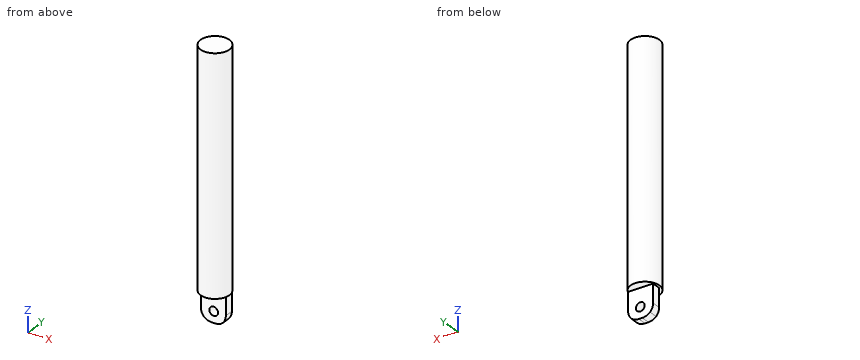
from build123d import *

# Parameters (mm, degrees)
SKETCH1_W           = 80
SKETCH1_H           = 4.95
SKETCH2_W           = 8.501628875
SKETCH2_H           = 3.058191312
BOSS_EXTRUDE1_DEPTH = 50
CHAMFER1_SIZE       = 2
FILLET1_R           = 4
HOLE1_START         = -3.599264013
HOLE1_OUTLINE_R     = 1.5
HOLE1_DEPTH         = 3.058191312
SCALE1_SCALE        = 18.33


# Read off the part's stored shape, not the designer's step: Hole1
with BuildPart() as part:
    # Sketch1 → Revolve1 (revolve)
    with BuildSketch(Plane(origin=(0, 0, 0), x_dir=(0, 0, -1), z_dir=(1, 0, 0))):
        Rectangle(SKETCH1_W, SKETCH1_H)
    revolve(axis=Axis((0, -2.475, -40), (0, 0, 1)))

    # Sketch2 → Boss-Extrude1 (add)
    with BuildSketch(Plane.XY):
        with Locations((0.196159038, -2.070168357)):
            Rectangle(SKETCH2_W, SKETCH2_H)
    extrude(amount=-BOSS_EXTRUDE1_DEPTH)

    # Chamfer1
    chamfer1_edges = [part.edges().sort_by_distance(p)[0] for p in [
        (4.446973476, -2.070168357, -50),
        (-4.054655399, -2.070168357, -50),
    ]]
    chamfer(chamfer1_edges, length=CHAMFER1_SIZE)

    # Fillet1
    # the kernel refuses this fillet: 4 mm, written as the material it takes off along each edge
    with BuildSketch(Plane(origin=(-2.054655399, 3.601062923, -50), x_dir=(-0.7071067811865491, 0, 0.7071067811865459), z_dir=(0, -1, 0)), Plane(origin=(4.446973476, -7.741399637, -48), x_dir=(0, 0, 1), z_dir=(0, 1, 0)), Plane(origin=(-4.054655399, 3.601062923, -48), x_dir=(0, 0, 1), z_dir=(0, -1, 0))) as fillet1_piece_1:
        with BuildLine():
            CenterArc((FILLET1_R * 0.414213562373, -FILLET1_R), FILLET1_R, 90, 45)
            Line((-FILLET1_R * 0.292893218813, -FILLET1_R * 0.292893218813), (0, 0))
            Line((0, 0), (FILLET1_R * 0.414213562373, 0))
        make_face()
    extrude(amount=11.34246256, mode=Mode.SUBTRACT)
    with BuildSketch(Plane(origin=(2.446973476, -7.741399637, -50), x_dir=(-1, 0, 0), z_dir=(0, 1, 0))) as fillet1_piece_2:
        with BuildLine():
            CenterArc((FILLET1_R * 0.414213562373, FILLET1_R), FILLET1_R, 225, 45)
            Line((-FILLET1_R * 0.292893218813, FILLET1_R * 0.292893218813), (0, 0))
            Line((0, 0), (FILLET1_R * 0.414213562373, 0))
        make_face()
    extrude(amount=11.34246256, mode=Mode.SUBTRACT)

    # Hole1 outline → Hole1 (cut)
    with BuildSketch(Plane(origin=(0, 0, 0), x_dir=(1, 0, 0), z_dir=(0, 1, 0)).offset(HOLE1_START)):
        with Locations((0.316437215, 46.206035657)):
            Circle(HOLE1_OUTLINE_R)
    extrude(amount=HOLE1_DEPTH, mode=Mode.SUBTRACT)


with BuildPart() as part_1:
    # Scale1: scaled about (0.006416206, -2.460917228, -1.550485335)
    add(part.part.scale(SCALE1_SCALE).moved(Location((-0.11119285, 42.647695561, 26.869910856))))


solid = part_1.part
Can you work these out from the model? Positions are in its coordinate system, mm. Round coordinates to 2 decimals unless told otherwise and drop trailing zeros. Loops run counter-clockwise (first coordinate to the right, second up) from the corner with the lowest first, then second, coordinate; pieces in that order, holes last. Notation, with made-up numbers: (-13.5, 23) - (20.5, 23) arc R10 cw to (20.5, 38) - close; hole circle Ø6 at (33.5, -34.75). An arc over 180 degrees is marked (long way). Answer in a Markdown table with one row per item. Add a question column.
Q1. I want a section at D-D on z = -276.5. List the corners of the cut face in (x, y) for me.
Q2. I want a section at C-C on y = -57. List the corners of the cut face in (x, z) for me.
Q3. For pin 1 Ø10 at (x, z) = (-72, -262) entering from -Y; pin 2 Ø1.5 at (x, y) = (39.5, -44) entering from -Z; pin 3 Ø1.5 at (x, z) = (45, 363) entering from +Y, each with a flat end and sliding along its axis, tell me the tip position at first contact or that it passes through.
Q4. I want a section at B-B on x = -42. List the corners of the cut face in (y, z) for me, and give its area (3 significant figures).
Q5. I need wall thicknesses on L1, parallel to Z at x = 3, y = 21; L2, parallel to Z at x = 1.5, y = -11.5; L3, parallel to Z at x = 37.5, y = -27. Which ranges of each line are inside material? Lowest first, please.
Q6. I want a section at A-A on y = 7.5. List the corners of the cut face in (x, z) for me (3 decimals), and give its area (3 significant figures).
A:
| question | item | result |
|---|---|---|
| 1 | outline | circle Ø181.47 at (-0.11, -2.72) |
| 2 | outline | (-72.82, -706.33) - (72.59, -706.33) - (72.59, 760.07) - (-72.82, 760.07) - close |
| 3 | pin 1 | y = -64.03 |
| 3 | pin 2 | z = -706.33 |
| 3 | pin 3 | y = 76.43 |
| 4 | outline | (-83.2, -706.33) - (-23.33, -706.33) - (-23.33, -880.95) - (32.73, -880.95) - (32.73, -706.33) - (77.77, -706.33) - (77.77, 760.07) - (-83.2, 760.07) - close |
| 4 | area | 246,000 mm^2 |
| 5 | L1 | -889.63 to -847.45, -792.72 to 760.07 |
| 5 | L2 | -889.63 to -847.26, -792.91 to 760.07 |
| 5 | L3 | -706.33 to 760.07 |
| 6 | outline | (-90.267, -706.33) - (-74.433, -706.33) - (-74.433, -822.6) arc R73.32 ccw to (-56.008, -871.205) arc R73.32 ccw to (-7.403, -889.63) - (14.372, -889.63) arc R73.32 ccw to (62.976, -871.205) arc R73.32 ccw to (81.402, -822.6) - (81.402, -706.33) - (90.045, -706.33) - (90.045, 760.07) - (-90.267, 760.07) - close; hole circle Ø54.99 at (5.689, -820.087) |
| 6 | area | 289,000 mm^2 |
